Input: part model. Units: mm. Frame: model coordinates. A direction names the side the tool comes from. Give positions to 0.01 mm unless a question says otherwise; leave off trailing zeros. Write each loop counter-clockwise with the first axis right and the second up, starting at its lowest first coordinate (ties: lowest second). Pieces come first, ordered by that corner, then holes. Notation, with made-up numbers: (-22, 12) - (-18, 12) arc R8 cw to (-18, 23) - close; hole circle Ø1 at (0.5, 62). An arc over 180 degrees is marked (long way). Answer as CSV lines item,"result".
```python
from build123d import *

# Parameters (mm, degrees)
SKETCH_R        = 10
SKETCH_R_2      = 2.5
PAD_DEPTH       = 5
PAD_DEPTH_BACK  = 5
SKETCH001_W     = 9
SKETCH001_H     = 5.15
POCKET_DEPTH    = 16
CHAMFER_SIZE    = 0.5
FILLET_R        = 1.5
CHAMFER001_SIZE = 0.5
FILLET001_R     = 0.7


with BuildPart() as part:
    # Sketch → Pad (new body, two sides)
    with BuildSketch(Plane.XY) as pad_sk:
        Circle(SKETCH_R)
        Circle(SKETCH_R_2, mode=Mode.SUBTRACT)
    extrude(amount=PAD_DEPTH)
    extrude(pad_sk.sketch, amount=-PAD_DEPTH_BACK)

    # Sketch001 (on DatumPlane) → Pocket (cut)
    with BuildSketch(Plane.YZ.offset(10)):
        Rectangle(SKETCH001_W, SKETCH001_H)
    extrude(amount=-POCKET_DEPTH, mode=Mode.SUBTRACT)

    # Chamfer
    chamfer_edges = [part.edges().sort_by_distance(p)[0] for p in [
        (-2.5, 0, -5),
        (-2.5, 0, 2.575),
    ]]
    chamfer(chamfer_edges, length=CHAMFER_SIZE)

    # Fillet
    fillet_edges = [part.edges().sort_by_distance(p)[0] for p in [
        (-6, 0, 2.575),
        (-6, 4.5, 0),
        (-6, 0, -2.575),
        (-6, -4.5, 0),
    ]]
    fillet(fillet_edges, radius=FILLET_R)

    # Chamfer001
    chamfer001_edges = [part.edges().sort_by_distance(p)[0] for p in [
        (9.728897, -2.312698, -2.575),
        (8.930286, -4.5, 0),
        (9.728897, -2.312698, 2.575),
        (9.728897, 2.312698, 2.575),
        (8.930286, 4.5, 0),
        (9.728897, 2.312698, -2.575),
    ]]
    chamfer(chamfer001_edges, length=CHAMFER001_SIZE)

    # Fillet001
    fillet001_edges = [part.edges().sort_by_distance(p)[0] for p in [
        (-10, 0, 5),
        (-10, 0, -5),
    ]]
    fillet(fillet001_edges, radius=FILLET001_R)


solid = part.part
```
Item 1: Reachability of faces 1 (the face through (-5.572, 0.063, -2.124)), 2 (the face through (4, 0, -5)) from +Z, -Z, +X, -X, +Y, -Y: full face, straight path, thin tool, end or side. Return the list, or none.
The answers:
face 1,"+X"
face 2,"-Z, +X, -X, +Y, -Y"
Item 2: Cut plane D-D on z = -1.75. Return the cut outline in (x, y) (3 decimals), plus the area to 3 significant figures.
The answers:
outline,"(-5.84, -3.675) - (-5.84, 3.675) arc R1.5 cw to (-4.5, 4.5) - (8.43, 4.5) - (8.694, 4.941) arc R10 ccw (long way) to (8.694, -4.941) - (8.43, -4.5) - (-4.5, -4.5) arc R1.5 cw to start"
area,"175 mm²"
Item 3: Cut plane C-C on z = 0. Return the cut outline in (x, y).
The answers:
outline,"(-6, -3) - (-6, 3) arc R1.5 cw to (-4.5, 4.5) - (8.43, 4.5) - (8.69, 4.94) arc R10 ccw (long way) to (8.69, -4.94) - (8.43, -4.5) - (-4.5, -4.5) arc R1.5 cw to start"
Item 4: Contact query for flat-ended pins moving along their axis: pin 1 (4 mm diameter, centred on x = 3, z = -1, fed in from -Y); pin 2 (6 mm diameter, centred on x = 6, z = -2, fed in from +Y); pin 3 (2.5 mm diameter, centred on y = -1.5, z = -0.5, fed in from +X). Output: stop coordinate, or through.
The answers:
pin 1,"y = -9.95"
pin 2,"y = 9.54"
pin 3,"x = -5.84"
Item 5: Ray query, line 1 (Z direction, x = 3, y = -0.25) (3 decimals); line 2 (Y direction, x = 0, z = 3.9); line 3 (Y direction, x = 7, z = -1.5). Return the intervals inside material, ascending. Write a range as from..to.
The answers:
line 1,"-5..-2.575, 2.575..5"
line 2,"-10..-2.5, 2.5..10"
line 3,"-7.14..-4.5, 4.5..7.14"
Item 6: Cut plane A-A on x = 0. Return the cut outline in (y, z) (3 decimals).
The answers:
outline,"(-10, -4.3) arc R0.7 ccw to (-9.3, -5) - (-3, -5) - (-2.5, -4.5) - (-2.5, -2.575) - (-4.5, -2.575) - (-4.5, 2.575) - (-3, 2.575) - (-2.5, 3.075) - (-2.5, 5) - (-9.3, 5) arc R0.7 ccw to (-10, 4.3) - close; (2.5, -4.5) - (3, -5) - (9.3, -5) arc R0.7 ccw to (10, -4.3) - (10, 4.3) arc R0.7 ccw to (9.3, 5) - (2.5, 5) - (2.5, 3.075) - (3, 2.575) - (4.5, 2.575) - (4.5, -2.575) - (2.5, -2.575) - close"
Item 7: Mould query, pull axis Y, two halves, no side actions, for faces 3 (the face through (-5.549, 0.063, 2.147)), 4 (the face through (-0.54, -2.44, -3.52)), 5 (the face through (-10, 0, 0)), 6 (the face through (2, -2, 5)). Classes: +Y half, -Y half, draft (parallel to the pull), parting line (faces both ways), or undercut.
The answers:
face 3,"undercut"
face 4,"undercut"
face 5,"parting line"
face 6,"draft"
Item 8: Cut plane B-B on y = 0. Return the cut outline in (x, z) (3 decimals).
The answers:
outline,"(-10, -4.3) arc R0.7 ccw to (-9.3, -5) - (-3, -5) - (-2.5, -4.5) - (-2.5, -2.575) - (-4.5, -2.575) arc R1.5 cw to (-6, -1.075) - (-6, 1.075) arc R1.5 cw to (-4.5, 2.575) - (-3, 2.575) - (-2.5, 3.075) - (-2.5, 5) - (-9.3, 5) arc R0.7 ccw to (-10, 4.3) - close; (2.5, -4.5) - (3, -5) - (9.3, -5) arc R0.7 ccw to (10, -4.3) - (10, -3.075) - (9.5, -2.575) - (2.5, -2.575) - close; (2.5, 3.075) - (3, 2.575) - (9.5, 2.575) - (10, 3.075) - (10, 4.3) arc R0.7 ccw to (9.3, 5) - (2.5, 5) - close"
